Work out the finished part from the listing and answer in its coordinate system (mm). Face numbers are marked on the shaded views. A direction names the side the tool comes from. Round coordinates to 2 decimals unless told otherwise and drop trailing zeros. Order: outer loops, then holes, each group sorted by start corner. A loop starts at its lowest first (then second) coordinate and runs counter-clockwise, first axis right, second up. Notation, with made-up numbers: (44, -10) - (69, -10) arc R29 cw to (69, 23) - close; hole circle Ø2 at (38, -27). An arc over 180 degrees is marked (long way). Use CSV: the item, a comma, the result in double quotes.
from build123d import *

# Parameters (mm, degrees)
BOSS_EXTRUDE1_DEPTH = 11.5
SKETCH1_13_R        = 1.5
SKETCH1_13_R_2      = 1.25
BOSS_EXTRUDE2_DEPTH = 7.75
BOSS_EXTRUDE3_DEPTH = 7
SKETCH2_W           = 23
SKETCH2_H           = 23
BOSS_EXTRUDE4_DEPTH = 190
SKETCH9_W           = 23.612347762
SKETCH9_H           = 7.954482618
CUT_EXTRUDE1_DEPTH  = 57
SKETCH8_W           = 57.001402056
SKETCH8_H           = 19.999995634
CUT_EXTRUDE5_DEPTH  = 11.5
SKETCH8_6_W         = 40.001402056
SKETCH8_6_H         = 19.999995634
SKETCH8_6_R         = 1.5
CUT_EXTRUDE7_DEPTH  = 15.55
SKETCH11_W          = 122.346056991
SKETCH11_H          = 8
CUT_EXTRUDE8_DEPTH  = 85.55
SKETCH10_W          = 122.346056991
SKETCH10_H          = 8
CUT_EXTRUDE9_DEPTH  = 105.55


with BuildPart() as part:
    # Sketch1 → Boss-Extrude1 (new, symmetric)
    with BuildSketch(Plane(origin=(0, 0, 0), x_dir=(1, 0, 0), z_dir=(0, 1, 0))):
        with BuildLine():
            Line((6.824314586, 7.284360201), (6.824314586, 9.00020274))
            Line((6.824314586, 9.00020274), (-3.690467309, 9.00020274))
            Line((-3.690467309, 9.00020274), (-17.038497557, 11.5))
            Line((-17.038497557, 11.5), (-24.867971487, 11.5))
            Line((-24.867971487, 11.5), (-24.867971487, -11.5))
            Line((-24.867971487, -11.5), (-17.038497557, -11.5))
            Line((-17.038497557, -11.5), (-3.690467309, -9.00020274))
            Line((-3.690467309, -9.00020274), (6.824314586, -9.00020274))
            Line((6.824314586, -9.00020274), (6.824314586, -7.284360201))
            ThreePointArc((6.824314586, -7.284360201), (4.861171432, -6.879883717), (3.082035449, -5.956732906))
            Line((3.082035449, -5.956732906), (-3.422402494, -3.8))
            Line((-3.422402494, -3.8), (-19.513448301, -3.98254267))
            Line((-19.513448301, -3.98254267), (-19.513448301, 3.8))
            Line((-19.513448301, 3.8), (-3.422402494, 3.8))
            Line((-3.422402494, 3.8), (3.082035449, 5.956732906))
            ThreePointArc((3.082035449, 5.956732906), (4.861171432, 6.879883717), (6.824314586, 7.284360201))
        make_face()
    extrude(amount=BOSS_EXTRUDE1_DEPTH, both=True)

    # Sketch1_13 → Boss-Extrude2 (add, symmetric)
    with BuildSketch(Plane(origin=(0, 0, 0), x_dir=(1, 0, 0), z_dir=(0, 1, 0))):
        with BuildLine():
            Line((6.824314586, 3.971385595), (6.824314586, 7.284360201))
            ThreePointArc((6.824314586, 7.284360201), (4.861171432, 6.879883717), (3.082035449, 5.956732906))
            Line((3.082035449, 5.956732906), (-3.422402494, 3.8))
            Line((-3.422402494, 3.8), (-19.513448301, 3.8))
            Line((-19.513448301, 3.8), (-19.513448301, -3.98254267))
            Line((-19.513448301, -3.98254267), (-3.422402494, -3.8))
            Line((-3.422402494, -3.8), (3.082035449, -5.956732906))
            ThreePointArc((3.082035449, -5.956732906), (4.861171432, -6.879883717), (6.824314586, -7.284360201))
            Line((6.824314586, -7.284360201), (6.824314586, -3.971385595))
            ThreePointArc((6.824314586, -3.971385595), (3.301909035, 0), (6.824314586, 3.971385595))
        make_face()
        with Locations(Location((-17.038497557, 0, 0), (0, 0, 270))):
            Circle(SKETCH1_13_R, mode=Mode.SUBTRACT)
        with Locations(Location((-13.038497557, 0, 0), (0, 0, 270))):
            Circle(SKETCH1_13_R, mode=Mode.SUBTRACT)
        with Locations(Location((-2.172402494, 0, 0), (0, 0, 270))):
            Circle(SKETCH1_13_R_2, mode=Mode.SUBTRACT)
    extrude(amount=BOSS_EXTRUDE2_DEPTH, both=True)

    # Sketch1_14 → Boss-Extrude3 (add, symmetric)
    with BuildSketch(Plane(origin=(0, 0, 0), x_dir=(1, 0, 0), z_dir=(0, 1, 0))):
        with BuildLine():
            Line((6.824314586, -3.971385595), (6.824314586, 3.971385595))
            ThreePointArc((6.824314586, 3.971385595), (3.301909035, 0), (6.824314586, -3.971385595))
        make_face()
    extrude(amount=BOSS_EXTRUDE3_DEPTH, both=True)

    # Sketch2 → Boss-Extrude4 (add)
    with BuildSketch(Plane.ZY.offset(24.867971487)):
        Rectangle(SKETCH2_W, SKETCH2_H)
    extrude(amount=BOSS_EXTRUDE4_DEPTH)

    # Sketch9 → Cut-Extrude1 (cut)
    with BuildSketch(Plane.ZY.offset(214.867971487)):
        with Locations((-0.306173881, 7.522758691)):
            Rectangle(SKETCH9_W, SKETCH9_H)
    extrude(amount=-CUT_EXTRUDE1_DEPTH, mode=Mode.SUBTRACT)

    # Sketch8 → Cut-Extrude5 (cut)
    with BuildSketch(Plane.XZ.offset(11.5)):
        with Locations((-186.367270459, 2.183e-06)):
            Rectangle(SKETCH8_W, SKETCH8_H)
    extrude(amount=-CUT_EXTRUDE5_DEPTH, mode=Mode.SUBTRACT)

    # Sketch8_6 → Cut-Extrude7 (cut)
    with BuildSketch(Plane.XZ.offset(11.5)):
        with Locations((-186.367270459, 2.183e-06)):
            Rectangle(SKETCH8_6_W, SKETCH8_6_H)
        with Locations(Location((-210.617971487, 5.162283196, 0), (0, 0, 270))):
            Circle(SKETCH8_6_R)
        with Locations(Location((-210.439498104, -5.010019091, 0), (0, 0, 270))):
            Circle(SKETCH8_6_R)
        with Locations(Location((-162.116569431, 5.124855295, 0), (0, 0, 270))):
            Circle(SKETCH8_6_R)
        with Locations(Location((-162.171918624, -5.125135232, 0), (0, 0, 270))):
            Circle(SKETCH8_6_R)
    extrude(amount=-CUT_EXTRUDE7_DEPTH, mode=Mode.SUBTRACT)

    # Sketch11 → Cut-Extrude8 (cut)
    with BuildSketch(Plane.XY.offset(11.5)):
        with Locations((-88.686476797, 0)):
            Rectangle(SKETCH11_W, SKETCH11_H)
    extrude(amount=-CUT_EXTRUDE8_DEPTH, mode=Mode.SUBTRACT)

    # Sketch10 → Cut-Extrude9 (cut)
    with BuildSketch(Plane(origin=(0, 11.5, 0), x_dir=(1, 0, 0), z_dir=(0, 1, 0))):
        with Locations((-88.686476797, 0.01745733)):
            Rectangle(SKETCH10_W, SKETCH10_H)
    extrude(amount=-CUT_EXTRUDE9_DEPTH, mode=Mode.SUBTRACT)


solid = part.part
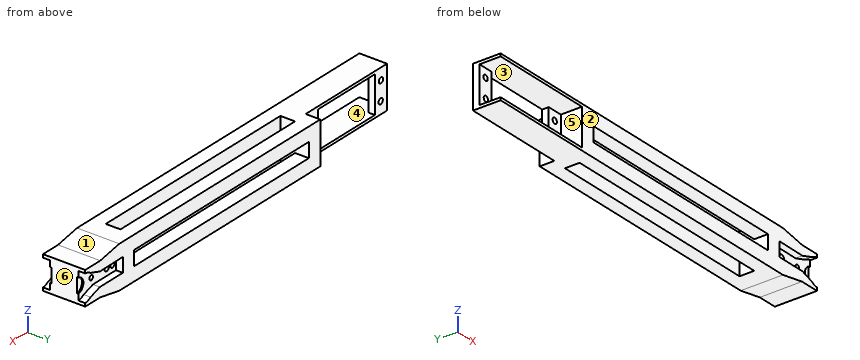
(1) For the marked faces 5 and 6, determine the directions among +Z, -Z, +X, -X, +Y, -Y from which every point of the face is accessible in a straight line to the end or side of a thin tool.
Findings below:
face 5,"-X, -Y"
face 6,"+Z, -Z, +X, +Y, -Y"
(2) Find section A-A (x = -196). Determine the outline of the cut face in (y, z).
Findings below:
outline,"(-11.5, -11.5) - (3.55, -11.5) - (3.55, -10) - (-11.5, -10) - close; (-11.5, 10) - (3.55, 10) - (3.55, 11.5) - (-11.5, 11.5) - close"
(3) Find the intervals of material crossed by L1, parallel to X at y = -2.5, z = 0; L2, parallel to X at y = 4.75, z = 0.25; L3, parallel to X at y = 0.75, z = 8, in increasing order. Write a range as from..to.
Findings below:
L1,"x = -157.87..-149.86, -27.51..-18.54, -15.54..-14.54, -11.54..-3.42, -0.92..6.82"
L2,"x = -157.87..-149.86, -27.51..-18.52, -15.56..-14.52, -11.56..-3.4, -0.95..6.82"
L3,"x = -214.87..-206.37, -166.37..-149.86, -27.51..6.82"
(4) Each of these flat-tipped pins is pushed along its axis until it touches: pin 1 (1.1 mm diameter, centred on y = -9.5, z = 1.5, fed in from +X); pin 2 (1 mm diameter, centred on y = -1, z = -9, fed in from -X); pin 3 (2.5 mm diameter, centred on x = -210.62, z = 5.16, fed in from -Y); pin 4 (1.8 mm diameter, centred on x = 5, z = -1.5, fed in from -Y). Where does it stop, or does it pass through?
Findings below:
pin 1,"stops at x = -19.51"
pin 2,"stops at x = -157.87"
pin 3,"passes through"
pin 4,"stops at y = -7"
(5) Find section B-B (x = -69.5). Determine the outline of the cut face in (y, z).
Findings below:
outline,"(-11.5, -11.5) - (-4, -11.5) - (-4, -4.02) - (-11.5, -4.02) - close; (-11.5, 3.98) - (-4, 3.98) - (-4, 11.5) - (-11.5, 11.5) - close; (4, -11.5) - (11.5, -11.5) - (11.5, -4.02) - (4, -4.02) - close; (4, 3.98) - (11.5, 3.98) - (11.5, 11.5) - (4, 11.5) - close"
(6) The mould has two halves that part along Z. Classify the marked faces 1, 2, 3 and 4: released by +Z, released by -Z, zero draft, split by the parting line, or undercut.
Findings below:
face 1,"released by +Z"
face 2,"zero draft"
face 3,"undercut"
face 4,"undercut"
